```python
from build123d import *

# Parameters (mm, degrees)
F0_R     = 190.5
F0_R_2   = 12.7
F0_R_3   = 101.6
F1_DEPTH = 39.624
F2_R     = 130.175
F2_R_2   = 101.6
F3_DEPTH = 3.175
F4_R     = 2.54


with BuildPart() as f1:
    # F0 (on Front) → F1 (new body)
    with BuildSketch(Plane.XZ):
        Circle(F0_R)
        with Locations((-116.74333, -116.74333)):
            Circle(F0_R_2, mode=Mode.SUBTRACT)
        with Locations((-42.731024, -159.474354)):
            Circle(F0_R_2, mode=Mode.SUBTRACT)
        with Locations((-159.474354, -42.731024)):
            Circle(F0_R_2, mode=Mode.SUBTRACT)
        with Locations((42.731024, -159.474354)):
            Circle(F0_R_2, mode=Mode.SUBTRACT)
        with Locations((116.74333, -116.74333)):
            Circle(F0_R_2, mode=Mode.SUBTRACT)
        with Locations((159.474354, -42.731024)):
            Circle(F0_R_2, mode=Mode.SUBTRACT)
        with Locations((-159.474354, 42.731024)):
            Circle(F0_R_2, mode=Mode.SUBTRACT)
        with Locations((-116.74333, 116.74333)):
            Circle(F0_R_2, mode=Mode.SUBTRACT)
        with Locations((-42.731024, 159.474354)):
            Circle(F0_R_2, mode=Mode.SUBTRACT)
        Circle(F0_R_3, mode=Mode.SUBTRACT)
        with Locations((159.474354, 42.731024)):
            Circle(F0_R_2, mode=Mode.SUBTRACT)
        with Locations((42.731024, 159.474354)):
            Circle(F0_R_2, mode=Mode.SUBTRACT)
        with Locations((116.74333, 116.74333)):
            Circle(F0_R_2, mode=Mode.SUBTRACT)
    extrude(amount=F1_DEPTH)

    # F2 (on face) → F3 (join)
    with BuildSketch(Plane.XZ.offset(39.624)):
        Circle(F2_R)
        Circle(F2_R_2, mode=Mode.SUBTRACT)
    extrude(amount=F3_DEPTH)

    # F4
    f4_edges = [f1.edges().sort_by_distance(p)[0] for p in [
        (-190.5, -39.624, 0),
        (-190.5, 0, 0),
        (-130.175, -39.624, 0),
    ]]
    fillet(f4_edges, radius=F4_R)


solid = f1.part
```
Geometry check sheet. Reference: the model listing, model coordinates, mm. A direction names the side the tool comes from. Round coordinates to 2 decimals unless told otherwise and drop trailing zeros. Loops run counter-clockwise (first coordinate to the right, second up) from the corner with the lowest first, then second, coordinate; pieces in that order, holes last. Notation, with made-up numbers: (27, 81.5) - (52, 81.5) arc R21 cw to (52, 104.5) - close; hole circle Ø2 at (63, 41). An arc over 180 degrees is marked (long way). Write item = value, one per line. Start each with the question number.
1. Mould release check, pull along Z, two halves, no side actions. Record for faces 3 (the face through (-110.88, -19.53, 105.48)), 4 (the face through (-151.17, -19.57, -115.92)), 5 (the face through (81, 0, -81)), 6 (the face through (-147.743, -19.535, -47.595)): released by +Z, released by -Z, zero draft, split by the parting line, or undercut.
2. Section check A-A on z = 0. Enter the section's corners in (x, y) (3 decimals), then the cut area to 3 significant figures.
3. Depth check by flat-ended pin: pin 1 (23 mm diameter, centred on x = 159.47, z = 42.73, fed in from -Y); pin 2 (3 mm diameter, centred on y = -36, z = 130.5, fed in from -X); pin 3 (3 mm diameter, centred on x = 11, z = 112.5, fed in from +Y); pin 4 (4 mm diameter, centred on y = -23, z = 87, fed in from +X). Enter the tip coordinate at first touch or a pass-through.
4. Thickness scan on line 1 (Z direction, x = -37, y = -2); line 2 (X direction, y = -39, z = -166); line 3 (Z direction, x = 52.5, y = -26). Record the ranges inside material, lowest first.
5. Section check C-C on y = -7.5. Give the number of separate pieces and of enclosed holes in the cut face, then the cut area to 3 significant figures.
6. Set-up check for faces 1 (the face through (-103.3, -42.48, -79.21)), 2 (the face through (171.206, -19.535, -47.595)): record each of +Z, -Z, +X, -X, +Y, -Y from which the full face is reachable in a straight line by a thin tool's end or side.
7. Section check B-B on x = 0. Enter the section's corners in (y, z) (3 decimals), then the cut area to 3 significant figures.
Working result:
q1.face_3 = undercut
q1.face_4 = split by the parting line
q1.face_5 = zero draft
q1.face_6 = undercut
q2.outline = (-190.5, -37.084) arc R2.54 ccw to (-187.96, -39.624) - (-132.715, -39.624) arc R2.54 cw to (-130.175, -42.164) - (-130.175, -42.799) - (-101.6, -42.799) - (-101.6, 0) - (-187.96, 0) arc R2.54 ccw to (-190.5, -2.54) - close; (101.6, -42.799) - (130.175, -42.799) - (130.175, -42.164) arc R2.54 cw to (132.715, -39.624) - (187.96, -39.624) arc R2.54 ccw to (190.5, -37.084) - (190.5, -2.54) arc R2.54 ccw to (187.96, 0) - (101.6, 0) - close
q2.area = 7,220 mm^2
q3.pin_1 = through
q3.pin_2 = -140.18
q3.pin_3 = 0
q3.pin_4 = 170.49
q4.line_1 = -186.81 to -170.81, -148.14 to -94.62, 94.62 to 148.14, 170.81 to 186.81
q4.line_2 = -91.67 to -53.63, -31.84 to 31.84, 53.63 to 91.67
q4.line_3 = -183.12 to -167.59, -151.36 to -86.98, 86.98 to 151.36, 167.59 to 183.12
q5.separate_pieces = 1
q5.enclosed_holes = 13
q5.area = 75,500 mm^2
q6.face_1 = -Y
q6.face_2 = +Y, -Y
q7.outline = (-42.799, -130.175) - (-42.164, -130.175) arc R2.54 cw to (-39.624, -132.715) - (-39.624, -187.96) arc R2.54 ccw to (-37.084, -190.5) - (-2.54, -190.5) arc R2.54 ccw to (0, -187.96) - (0, -101.6) - (-42.799, -101.6) - close; (-42.799, 101.6) - (0, 101.6) - (0, 187.96) arc R2.54 ccw to (-2.54, 190.5) - (-37.084, 190.5) arc R2.54 ccw to (-39.624, 187.96) - (-39.624, 132.715) arc R2.54 cw to (-42.164, 130.175) - (-42.799, 130.175) - close
q7.area = 7,220 mm^2
